from build123d import *

# Parameters (mm, degrees)
SKETCH_W     = 302
SKETCH_H     = 112
SKETCH_W_2   = 287
SKETCH_H_2   = 97
PAD_DEPTH    = 4
SKETCH001_W  = 13
SKETCH001_H  = 7.5
POCKET_DEPTH = 4
FILLET_R     = 1
FILLET001_R  = 1
FILLET002_R  = 1
FILLET003_R  = 1
FILLET004_R  = 1
FILLET005_R  = 1
FILLET006_R  = 1
FILLET007_R  = 1
FILLET008_R  = 1
FILLET009_R  = 1
FILLET010_R  = 1
FILLET011_R  = 1


with BuildPart() as part:
    # Sketch → Pad (new body)
    with BuildSketch(Plane.XY):
        Rectangle(SKETCH_W, SKETCH_H)
        Rectangle(SKETCH_W_2, SKETCH_H_2, mode=Mode.SUBTRACT)
    extrude(amount=PAD_DEPTH)

    # Sketch001 (on Face10 of Pad) → Pocket (cut)
    with BuildSketch(Plane.XY.offset(4)):
        with Locations((-124, 52.25)):
            Rectangle(SKETCH001_W, SKETCH001_H)
    extrude(amount=-POCKET_DEPTH, mode=Mode.SUBTRACT)

    # Fillet
    fillet_edges = [part.edges().sort_by_distance(p)[0] for p in [
        (-130.5, 48.5, 2),
    ]]
    fillet(fillet_edges, radius=FILLET_R)

    # Fillet001
    fillet001_edges = [part.edges().sort_by_distance(p)[0] for p in [
        (-143.5, 48.5, 2),
    ]]
    fillet(fillet001_edges, radius=FILLET001_R)

    # Fillet002
    fillet002_edges = [part.edges().sort_by_distance(p)[0] for p in [
        (-117.5, 48.5, 2),
    ]]
    fillet(fillet002_edges, radius=FILLET002_R)

    # Fillet003
    fillet003_edges = [part.edges().sort_by_distance(p)[0] for p in [
        (-151, -56, 2),
    ]]
    fillet(fillet003_edges, radius=FILLET003_R)

    # Fillet004
    fillet004_edges = [part.edges().sort_by_distance(p)[0] for p in [
        (151, -56, 2),
    ]]
    fillet(fillet004_edges, radius=FILLET004_R)

    # Fillet005
    fillet005_edges = [part.edges().sort_by_distance(p)[0] for p in [
        (151, 56, 2),
    ]]
    fillet(fillet005_edges, radius=FILLET005_R)

    # Fillet006
    fillet006_edges = [part.edges().sort_by_distance(p)[0] for p in [
        (-117.5, 56, 2),
    ]]
    fillet(fillet006_edges, radius=FILLET006_R)

    # Fillet007
    fillet007_edges = [part.edges().sort_by_distance(p)[0] for p in [
        (-151, 56, 2),
    ]]
    fillet(fillet007_edges, radius=FILLET007_R)

    # Fillet008
    fillet008_edges = [part.edges().sort_by_distance(p)[0] for p in [
        (143.5, -48.5, 2),
    ]]
    fillet(fillet008_edges, radius=FILLET008_R)

    # Fillet009
    fillet009_edges = [part.edges().sort_by_distance(p)[0] for p in [
        (-143.5, -48.5, 2),
    ]]
    fillet(fillet009_edges, radius=FILLET009_R)

    # Fillet010
    fillet010_edges = [part.edges().sort_by_distance(p)[0] for p in [
        (143.5, 48.5, 2),
    ]]
    fillet(fillet010_edges, radius=FILLET010_R)

    # Fillet011
    fillet011_edges = [part.edges().sort_by_distance(p)[0] for p in [
        (-130.5, 56, 2),
    ]]
    fillet(fillet011_edges, radius=FILLET011_R)


solid = part.part
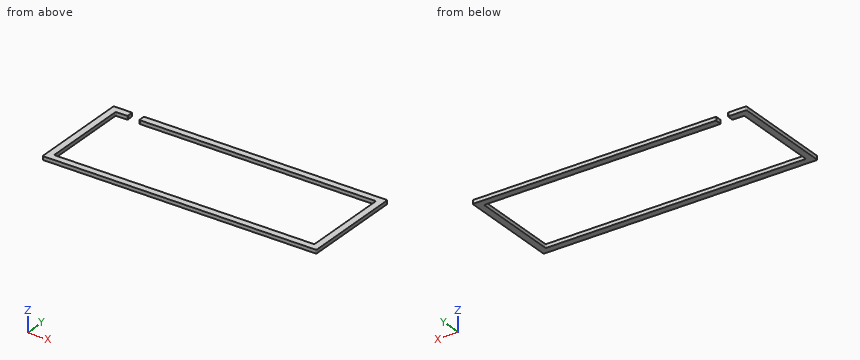
Can you work these out from the model? Positions are in its coordinate system, mm. Round coordinates to 2 decimals unless told otherwise and drop trailing zeros. Loops run counter-clockwise (first coordinate to the right, second up) from the corner with the lowest first, then second, coordinate; pieces in that order, holes last. Notation, with made-up numbers: (29, 30) - (87, 30) arc R3 ccw to (87, 35) - close; hole circle Ø8 at (80.5, -39). An arc over 180 degrees is marked (long way). Answer in a Markdown table with one row per item. Add a question column.
Q1. I want a section at A-A on x = 129. List the corners of the cut face in (y, z) for me.
Q2. I need wall thicknesses on L1, parallel to Y at x = 101.5, z = 1.5; L2, parallel to X at y = 26, z = 0.8; L3, parallel to X at y = 49, z = 1.4. Which ranges of each line are inside material? Lowest first, please.
Q3. I want a section at B-B on y = 36. List the corners of the cut face in (x, z) for me.
Q4. I want a section at C-C on z = 1.5. List the corners of the cut face in (x, y) for me.
A:
| question | item | result |
|---|---|---|
| 1 | outline | (-56, 0) - (-48.5, 0) - (-48.5, 4) - (-56, 4) - close; (48.5, 0) - (56, 0) - (56, 4) - (48.5, 4) - close |
| 2 | L1 | -56 to -48.5, 48.5 to 56 |
| 2 | L2 | -151 to -143.5, 143.5 to 151 |
| 2 | L3 | -151 to -130.63, -117.37 to 151 |
| 3 | outline | (-151, 0) - (-143.5, 0) - (-143.5, 4) - (-151, 4) - close; (143.5, 0) - (151, 0) - (151, 4) - (143.5, 4) - close |
| 4 | outline | (-151, -55) arc R1 ccw to (-150, -56) - (150, -56) arc R1 ccw to (151, -55) - (151, 55) arc R1 ccw to (150, 56) - (-116.5, 56) arc R1 ccw to (-117.5, 55) - (-117.5, 49.5) arc R1 ccw to (-116.5, 48.5) - (142.5, 48.5) arc R1 cw to (143.5, 47.5) - (143.5, -47.5) arc R1 cw to (142.5, -48.5) - (-142.5, -48.5) arc R1 cw to (-143.5, -47.5) - (-143.5, 47.5) arc R1 cw to (-142.5, 48.5) - (-131.5, 48.5) arc R1 ccw to (-130.5, 49.5) - (-130.5, 55) arc R1 ccw to (-131.5, 56) - (-150, 56) arc R1 ccw to (-151, 55) - close |
